Work out the finished part from the listing and answer in its coordinate system (mm). Face numbers are marked on the shaded views. A direction names the side the tool comes from. Give positions to 0.01 mm unless a question says otherwise; leave off trailing zeros. Order: outer loops, then holes, each group sorted by start corner. A loop starts at its lowest first (then second) coordinate and runs counter-clockwise, first axis right, second up. Notation, with made-up numbers: (-28.5, 70) -> (-10.5, 70) arc R15 ccw to (-10.5, 93) -> close; hole circle Ø2 at (6, -36.5). An arc over 180 degrees is marked (long way). Use a Markdown table: item, result. Add a question column.
```python
from build123d import *

# Parameters (mm, degrees)
BOSS_EXTRUDE1_DEPTH  = 3.175
EXTRUDE_THIN1_START  = -6.1722
EXTRUDE_THIN1_DEPTH  = 6.1722
BOSS_EXTRUDE2_DEPTH  = 2.9972
FILLET1_R            = 3.175
FILLET1_OF_MIRROR1_R = 3.175
BOSS_EXTRUDE3_START  = -6.1722
BOSS_EXTRUDE3_DEPTH  = 6.1722


with BuildPart() as part:
    # Sketch1 → Boss-Extrude1 (new body)
    with BuildSketch(Plane.ZY.offset(-35.1028)):
        with BuildLine():
            Line((-114.3, 38.1), (-114.3, -38.1))
            Line((-114.3, -38.1), (-184.15, -38.1))
            ThreePointArc((-184.15, -38.1), (-188.640128061, -36.240128061), (-190.5, -31.75))
            Line((-190.5, -31.75), (-190.5, 31.75))
            ThreePointArc((-190.5, 31.75), (-188.640128061, 36.240128061), (-184.15, 38.1))
            Line((-184.15, 38.1), (-114.3, 38.1))
        make_face()
    extrude(amount=BOSS_EXTRUDE1_DEPTH)

    # Sketch4 → Extrude-Thin1 (add)
    with BuildSketch(Plane.ZY.offset(-31.9278).offset(EXTRUDE_THIN1_START)):
        with BuildLine():
            Line((-114.3, 38.1), (-184.15, 38.1))
            ThreePointArc((-184.15, 38.1), (-188.640128061, 36.240128061), (-190.5, 31.75))
            Line((-190.5, 31.75), (-190.5, -31.75))
            ThreePointArc((-190.5, -31.75), (-188.640128061, -36.240128061), (-184.15, -38.1))
            Line((-184.15, -38.1), (-114.3, -38.1))
            Line((-114.3, -38.1), (-114.3, -40.64))
            Line((-114.3, -40.64), (-184.15, -40.64))
            ThreePointArc((-184.15, -40.64), (-190.436179285, -38.036179285), (-193.04, -31.75))
            Line((-193.04, -31.75), (-193.04, 31.75))
            ThreePointArc((-193.04, 31.75), (-190.436179285, 38.036179285), (-184.15, 40.64))
            Line((-184.15, 40.64), (-114.3, 40.64))
            Line((-114.3, 40.64), (-114.3, 38.1))
        make_face()
    extrude(amount=EXTRUDE_THIN1_DEPTH)

    # Sketch5 → Boss-Extrude2 (add)
    with BuildSketch(Plane.ZY.offset(-31.9278)):
        with BuildLine():
            Line((-177.8, 15.875), (-171.45, 15.875))
            Line((-171.45, 15.875), (-170.350147737, 15.24))
            Line((-170.350147737, 15.24), (-128.099852263, 15.24))
            Line((-128.099852263, 15.24), (-127, 15.875))
            Line((-127, 15.875), (-120.65, 15.875))
            ThreePointArc((-120.65, 15.875), (-117.475, 12.7), (-120.65, 9.525))
            Line((-120.65, 9.525), (-127, 9.525))
            Line((-127, 9.525), (-128.099852263, 10.16))
            Line((-128.099852263, 10.16), (-170.350147737, 10.16))
            Line((-170.350147737, 10.16), (-171.45, 9.525))
            Line((-171.45, 9.525), (-177.8, 9.525))
            ThreePointArc((-177.8, 9.525), (-180.975, 12.7), (-177.8, 15.875))
        make_face()
    boss_extrude2 = extrude(amount=BOSS_EXTRUDE2_DEPTH)

    # Fillet1
    fillet1_edges = [part.edges().sort_by_distance(p)[0] for p in [
        (30.4292, 15.875, -171.45),
        (30.4292, 9.525, -171.45),
        (30.4292, 9.525, -127),
        (30.4292, 15.875, -127),
    ]]
    fillet(fillet1_edges, radius=FILLET1_R)

    # Mirror1: Boss-Extrude2 across plane
    add(boss_extrude2.mirror(Plane.ZX))

    # Fillet1 of Mirror1
    fillet1_of_mirror1_edges = [part.edges().sort_by_distance(p)[0] for p in [
        (30.4292, -15.875, -171.45),
        (30.4292, -9.525, -171.45),
        (30.4292, -9.525, -127),
        (30.4292, -15.875, -127),
    ]]
    fillet(fillet1_of_mirror1_edges, radius=FILLET1_OF_MIRROR1_R)

    # Sketch6 → Boss-Extrude3 (add)
    with BuildSketch(Plane.ZY.offset(-31.9278).offset(BOSS_EXTRUDE3_START)):
        with BuildLine():
            Line((-193.04, 53.34), (-193.04, 31.75))
            ThreePointArc((-193.04, 31.75), (-190.436179285, 38.036179285), (-184.15, 40.64))
            Line((-184.15, 40.64), (-159.749231637, 40.64))
            ThreePointArc((-159.749231637, 40.64), (-164.609311228, 41.606729937), (-168.729487758, 44.359743879))
            Line((-168.729487758, 44.359743879), (-182.199871939, 57.830128061))
            ThreePointArc((-182.199871939, 57.830128061), (-189.120039796, 59.206635031), (-193.04, 53.34))
        make_face()
    extrude(amount=BOSS_EXTRUDE3_DEPTH)


solid = part.part
```
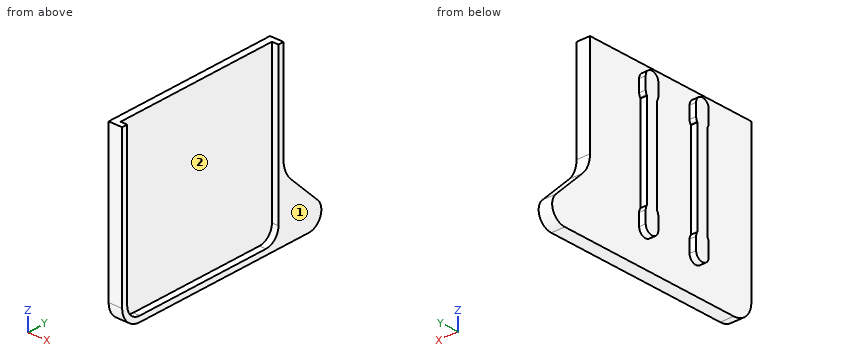
1) The part is cut by section A-A, the plane x = 33.25. Determine the outline of the cut face in (y, z).
2) Straight lines are drawn through the part: line 1 (Y direction, x = 30.5, z = -164.5); line 2 (Y direction, x = 29.5, z = -176.5) (3 decimals); line 3 (X direction, y = 37.5, z = -122). For each, find the intervals that lie inside material, in ascending order.
3) Flat-ended cylindrical pins translate along their axes: pin 1 (1.9 mm diameter, centred on x = 36.5, z = -130.5, fed in from +Y); pin 2 (1.5 mm diameter, centred on x = 30, z = -174, fed in from +Y) (3 decimals); pin 3 (0.9 mm diameter, centred on x = 30, z = -123.5, fed in from -Y) (3 decimals). Find the tip coordinate at first contact, or state that the pin passes through.
4) Which of the six approach directions +Z, -Z, +X, -X, +Y, -Y give full straight-line access (tool end or side, diameter ignored) to the marked faces 1 and 2?
5) The part is cut by section B-B, the plane z = -131. Determine the outline of the cut face in (x, y).
6) The part is cut by section C-C, the plane y = -12.7. Determine the outline of the cut face in (x, z) (3 decimals), then the cut area to 3 significant figures.
7) The part is cut by section D-D, the plane y = 22. Determine the outline of the cut face in (x, z), then the cut area to 3 significant figures.
A:
| question | item | result |
|---|---|---|
| 1 | outline | (-40.64, -184.15) arc R8.89 ccw to (-31.75, -193.04) -> (53.34, -193.04) arc R6.35 ccw to (57.83, -182.2) -> (44.36, -168.73) arc R12.7 cw to (40.64, -159.75) -> (40.64, -114.3) -> (-40.64, -114.3) -> close |
| 2 | line 1 | -15.24 to -10.16, 10.16 to 15.24 |
| 2 | line 2 | -15.875 to -9.525, 9.525 to 15.875 |
| 2 | line 3 | 31.93 to 35.1 |
| 3 | pin 1 | y = 40.64 |
| 3 | pin 2 | y = 15.875 |
| 3 | pin 3 | y = -15.875 |
| 4 | face 1 | +Z, -Z, +X, +Y, -Y |
| 4 | face 2 | +Z, +X |
| 5 | outline | (28.93, -15.24) -> (31.93, -15.24) -> (31.93, -40.64) -> (38.1, -40.64) -> (38.1, -38.1) -> (35.1, -38.1) -> (35.1, 38.1) -> (38.1, 38.1) -> (38.1, 40.64) -> (31.93, 40.64) -> (31.93, 15.24) -> (28.93, 15.24) -> (28.93, 10.16) -> (31.93, 10.16) -> (31.93, -10.16) -> (28.93, -10.16) -> close |
| 6 | outline | (28.931, -180.975) -> (31.928, -180.975) -> (31.928, -193.04) -> (38.1, -193.04) -> (38.1, -190.5) -> (35.103, -190.5) -> (35.103, -114.3) -> (31.928, -114.3) -> (31.928, -117.475) -> (28.931, -117.475) -> close |
| 6 | area | 448 mm^2 |
| 7 | outline | (31.93, -193.04) -> (38.1, -193.04) -> (38.1, -190.5) -> (35.1, -190.5) -> (35.1, -114.3) -> (31.93, -114.3) -> close |
| 7 | area | 258 mm^2 |
